```python
from build123d import *

# Parameters (mm, degrees)
SKETCH_1_W          = 200
SKETCH_1_H          = 60
EXTRUDE_1_DEPTH     = 2
SKETCH_3_R          = 2.55
CUT_EXTRUDE_1_DEPTH = 105.422219858
CUT_EXTRUDE_2_DEPTH = 96.828733232


with BuildPart() as part:
    # 草图1 → 凸台-拉伸1 (new body)
    with BuildSketch(Plane(origin=(0, 0, 0), x_dir=(1, 0, 0), z_dir=(0, 1, 0))):
        Rectangle(SKETCH_1_W, SKETCH_1_H)
    extrude(amount=EXTRUDE_1_DEPTH)

    # 草图3 → 切除-拉伸1 (cut, through all)
    with BuildSketch(Plane(origin=(0, 2, 0), x_dir=(1, 0, 0), z_dir=(0, 1, 0))):
        Polygon((82.173464202, -20.771330594), (-77.826535798, -20.771330594), (-86.642884834, 30), (-100, 30), (-100, -30), (100, -30), (100, 30), (90.989813237, 30), align=None)
        with Locations(Location((-74.153372817, 24, 0), (0, 0, 270))):
            Circle(SKETCH_3_R)
        with Locations(Location((-70.731615422, 4.294884514, 0), (0, 0, 270))):
            Circle(SKETCH_3_R)
        with Locations(Location((-67.309858027, -15.410230973, 0), (0, 0, 270))):
            Circle(SKETCH_3_R)
        with Locations(Location((78.50030122, 24, 0), (0, 0, 270))):
            Circle(SKETCH_3_R)
        with Locations(Location((71.65678643, -15.410230973, 0), (0, 0, 270))):
            Circle(SKETCH_3_R)
        with Locations(Location((75.078543825, 4.294884514, 0), (0, 0, 270))):
            Circle(SKETCH_3_R)
    extrude(amount=-CUT_EXTRUDE_1_DEPTH, mode=Mode.SUBTRACT)

    # 草图4 → 切除-拉伸2 (cut, through all)
    with BuildSketch(Plane.XZ):
        Polygon((76.083674975, 20.771330594), (84.90002401, -30), (90.989813237, -30), (82.173464202, 20.771330594), align=None)
        Polygon((-86.642884834, -30), (-80.553095607, -30), (-71.736746572, 20.771330594), (-77.826535798, 20.771330594), align=None)
    extrude(amount=-CUT_EXTRUDE_2_DEPTH, mode=Mode.SUBTRACT)


solid = part.part
```
Verification items for the finished model (mm, model axes). Round coordinates to 2 decimals unless told otherwise and drop trailing zeros. Write each loop counter-clockwise with the first axis right and the second up, starting at its lowest first coordinate (ties: lowest second). Pieces come first, ordered by that corner, then holes.
1. Section check B-B on y = 1.25. Enter the section's corners in (x, z), plus the area to 3 significant figures.
2. Section check A-A on z = -24. Enter the section's corners in (x, y).
3. Scan lines: L1, parallel to Z at x = -67, y = 0.3; L2, parallel to X at y = 0.6, z = -6; L3, parallel to X at y = 1.1, z = -22. Record each from-to range of solid material in increasing order.
4. Section check C-C on z = -13. Enter the section's corners in (x, y), plus the area to 3 significant figures.
5. Section check D-D on z = 10.5. Enter the section's corners in (x, y).
6. Draft check along X on faces 1 (the cylindrical face through (77.607, 1.014, -4.627)), 2 (the flat face through (1, 2, -5)), 3 (the flat face through (-76.207, 0.986, -4.97)). Enter one of: +X half, -X half, draft (parallel to the pull), parting line (faces both ways), or undercut.
Answer:
1. outline: (-80.55, -30) - (84.9, -30) - (76.08, 20.77) - (-71.74, 20.77) - close; hole circle Ø5.1 at (-74.15, -24); hole circle Ø5.1 at (-70.73, -4.29); hole circle Ø5.1 at (-67.31, 15.41); hole circle Ø5.1 at (71.66, 15.41); hole circle Ø5.1 at (75.08, -4.29); hole circle Ø5.1 at (78.5, -24)
1. area: 7,830 mm2
2. outline: (-79.51, 0) - (-76.7, 0) - (-76.7, 2) - (-79.51, 2) - close; (-71.6, 0) - (75.95, 0) - (75.95, 2) - (-71.6, 2) - close; (81.05, 0) - (83.86, 0) - (83.86, 2) - (81.05, 2) - close
3. L1: z = -30 to 12.88, 17.94 to 20.77
3. L2: x = -76.39 to -72.63, -68.84 to 73.18, 76.97 to 80.73
3. L3: x = -79.16 to -75.74, -72.57 to 76.92, 80.08 to 83.51
4. outline: (-77.6, 0) - (81.95, 0) - (81.95, 2) - (-77.6, 2) - close
4. area: 319 mm2
5. outline: (-73.52, 0) - (77.87, 0) - (77.87, 2) - (-73.52, 2) - close
6. face 1: undercut
6. face 2: draft
6. face 3: -X half
